from build123d import *

# Parameters (mm, degrees)
SKETCH_W        = 24.681526
SKETCH_H        = 55.414013
PAD_DEPTH       = 13
SKETCH001_W     = 15.923566
SKETCH001_H     = 11.305732
POCKET_DEPTH    = 55.415013
SKETCH002_R     = 2.87618
POCKET001_DEPTH = 13.001
SKETCH003_W     = 24.574786
SKETCH003_H     = 11.309867
PAD001_DEPTH    = 35
SKETCH004_W     = 11.522993
SKETCH004_H     = 4.823732
PAD002_DEPTH    = 22
PAD003_DEPTH    = 2
SKETCH006_R     = 9.566685
PAD004_DEPTH    = 24
SKETCH007_R     = 3.828287
POCKET002_DEPTH = 24.001
SKETCH008_R     = 13.5012954455
PAD005_DEPTH    = 13
SKETCH009_R     = 5.871137
POCKET003_DEPTH = 26.001


with BuildPart() as part:
    # Sketch → Pad (new body)
    with BuildSketch(Plane.XY):
        with Locations((-0.318477, 1.2738855)):
            Rectangle(SKETCH_W, SKETCH_H)
    extrude(amount=PAD_DEPTH)

    # Sketch001 (on Face3 of Pad) → Pocket (cut, through all)
    with BuildSketch(Plane.XZ.offset(26.433121)):
        with Locations((-0.079613, 1.512745)):
            Rectangle(SKETCH001_W, SKETCH001_H)
    extrude(amount=-POCKET_DEPTH, mode=Mode.SUBTRACT)

    # Sketch002 (on Face8 of Pocket) → Pocket001 (cut, through all)
    with BuildSketch(Plane.XY.offset(13)):
        with Locations((0, -18.630573)):
            Circle(SKETCH002_R)
    extrude(amount=-POCKET001_DEPTH, mode=Mode.SUBTRACT)

    # Sketch003 (on Face8 of Pocket001) → Pad001 (join)
    with BuildSketch(Plane.XY.offset(13)):
        with Locations((-0.333364, 23.2805385)):
            Rectangle(SKETCH003_W, SKETCH003_H)
    extrude(amount=PAD001_DEPTH)

    # Sketch004 (on Face9 of Pad001) → Pad002 (join)
    with BuildSketch(Plane(origin=(-12.65924, 0, 0), x_dir=(0, -1, 0), z_dir=(-1, 0, 0))):
        with Locations((-23.1981075, 6.669861)):
            Rectangle(SKETCH004_W, SKETCH004_H)
    extrude(amount=PAD002_DEPTH)

    # Sketch005 → Pad003 (join, symmetric)
    with BuildSketch(Plane.XZ.offset(-23)):
        Polygon((-34.666348, 8.690443), (-12.38179, 57.716461), (-12.38179, 8.690443), align=None)
    extrude(amount=PAD003_DEPTH, both=True)

    # Sketch006 → Pad004 (join)
    with BuildSketch(Plane.XY):
        with Locations((-36.756073, 22.431417)):
            Circle(SKETCH006_R)
    extrude(amount=PAD004_DEPTH)

    # Sketch007 (on Face27 of Pad004) → Pocket002 (cut, through all)
    with BuildSketch(Plane.XY.offset(24)):
        with Locations((-36.786556, 22.589872)):
            Circle(SKETCH007_R)
    extrude(amount=-POCKET002_DEPTH, mode=Mode.SUBTRACT)

    # Sketch008 → Pad005 (join, symmetric)
    with BuildSketch(Plane.XZ.offset(-23)):
        with Locations((0, 52.938587)):
            Circle(SKETCH008_R)
    extrude(amount=PAD005_DEPTH, both=True)

    # Sketch009 (on Face31 of Pad005) → Pocket003 (cut, through all)
    with BuildSketch(Plane.XZ.offset(-10)):
        with Locations((0, 52.790291)):
            Circle(SKETCH009_R)
    extrude(amount=-POCKET003_DEPTH, mode=Mode.SUBTRACT)


solid = part.part
The listing builds one solid part. Answer for the finished solid, in the listing's coordinates (mm). A direction names the side the tool comes from. Round coordinates to 2 decimals unless told otherwise and drop trailing zeros. Write each loop counter-clockwise with the first axis right and the second up, starting at its lowest first coordinate (ties: lowest second). Pieces come first, ordered by that corner, then holes. Notation, with made-up numbers: (87.25, 22.25) - (114.25, 22.25) arc R13 ccw to (114.25, 26.25) - close; hole circle Ø7 at (11.5, -37). An arc over 180 degrees is marked (long way). Use a Markdown table: item, result. Add a question column.
1. Flat-ended cylindrical pins translate along their axes: P1, Ø1, axis at x = -3, z = 19.5, coming from the -Y side; P2, Ø12, axis at y = -13.5, z = 14.5, coming from the -X side; P3, Ø2, axis at x = 2, y = 16.5, coming from the +Z side. Find the tip coordinate at first contact, or state that the pin passes through.
2. The part is cut by section C-C (z = 49.5). Write down the section's boundary in (x, y), and give its area (3 significant figures).
3. The part is cut by section D-D (y = 4). Write down the section's boundary in (x, z), and give its area (3 significant figures).
4. The part is cut by section A-A (x = 0). Write down the section's boundary in (y, z), and give its area (3 significant figures).
5. For a pull along X with two mould halves and no side action, classify faces 6 (the face through (-21, 27, 9.082)), 7 (the face through (12.022, 1, 6)), 8 (the face through (6, 10, 50)) as +X half, -X half, draft (parallel to the pull), parting line (faces both ways), or undercut.
6. Consider line 1 (X direction, y = 16, z = 53); line 2 (Z direction, x = 0, y = 28); line 3 (Y direction, x = 0, z = 10.5). Determine where each line is inside the solid, lowest interval first.
7. The part is cut by section B-B (y = 24). Write down the section's boundary in (x, z), and give its area (3 significant figures).
8. A tool of negligible diameter and unlimited length cuts with its end or side. For faces 1 (the face through (-12.621, 19, 30)), 2 (the face through (-8.041, 1, 4)), 3 (the face through (7.26, 22.82, 64.32)), 4 (the face through (0, 28.981, 8)), 5 (the face through (11.954, 23, 30)), from which of +Z, -Z, +X, -X, +Y, -Y can it reach the whole face along a straight path? Write none if from no direction.
Reported:
| question | item | result |
|---|---|---|
| 1 | P1 | y = 17.63 |
| 1 | P2 | x = -12.66 |
| 1 | P3 | z = 66.4 |
| 2 | outline | (-16.12, 21) - (-13.06, 21) - (-13.06, 10) - (-4.86, 10) - (-4.86, 36) - (-13.06, 36) - (-13.06, 25) - (-16.12, 25) - close; (4.86, 10) - (13.06, 10) - (13.06, 36) - (4.86, 36) - close |
| 2 | area | 438 mm^2 |
| 3 | outline | (-12.66, 0) - (-8.04, 0) - (-8.04, 7.17) - (7.88, 7.17) - (7.88, 0) - (12.02, 0) - (12.02, 13) - (-12.66, 13) - close |
| 3 | area | 207 mm^2 |
| 4 | outline | (-26.43, 7.17) - (-21.51, 7.17) - (-21.51, 13) - (-26.43, 13) - close; (-15.75, 7.17) - (28.98, 7.17) - (28.98, 13) - (28.94, 13) - (28.94, 39.44) - (36, 39.44) - (36, 46.92) - (10, 46.92) - (10, 39.44) - (17.63, 39.44) - (17.63, 13) - (-15.75, 13) - close; (10, 58.66) - (36, 58.66) - (36, 66.44) - (10, 66.44) - close |
| 4 | area | 986 mm^2 |
| 5 | face 6 | undercut |
| 5 | face 7 | +X half |
| 5 | face 8 | draft |
| 6 | line 1 | -13.5 to -5.87, 5.87 to 13.5 |
| 6 | line 2 | 7.17 to 46.92, 58.66 to 66.44 |
| 6 | line 3 | -26.43 to -21.51, -15.75 to 28.98 |
| 7 | outline | (-46.19, 0) - (-40.35, 0) - (-40.35, 24) - (-46.19, 24) - close; (-33.23, 0) - (-27.32, 0) - (-27.32, 4.26) - (-12.66, 4.26) - (-12.66, 0) - (-8.04, 0) - (-8.04, 7.17) - (7.88, 7.17) - (7.88, 0) - (12.02, 0) - (12.02, 13) - (11.95, 13) - (11.95, 46.66) arc R13.5 ccw (long way) to (-13.14, 56.06) - (-27.71, 24) - (-33.23, 24) - close; hole circle Ø11.74 at (0, 52.79) |
| 7 | area | 2,190 mm^2 |
| 8 | face 1 | -Y |
| 8 | face 2 | -Z, +Y, -Y |
| 8 | face 3 | none |
| 8 | face 4 | -Z, +X, +Y |
| 8 | face 5 | +X, +Y, -Y |
